Geometry: final body of the model. Coordinates: model frame, mm. Coordinates: 2 decimals unless noted, no trailing zeros. Write each loop counter-clockwise with the first axis right and the second up, starting at its lowest first coordinate (ties: lowest second). Pieces come first, ordered by that corner, then holes.
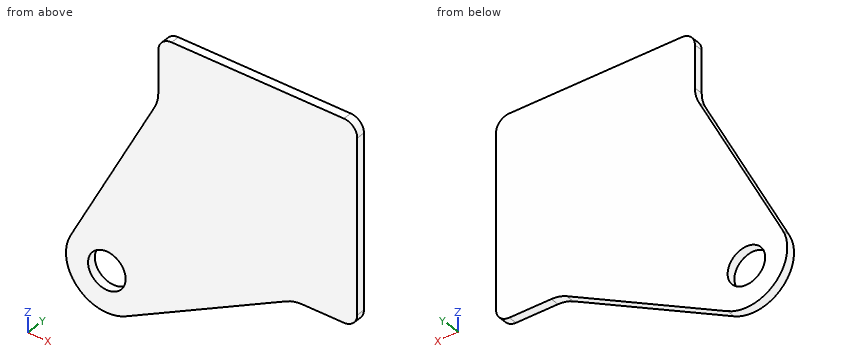
Autodesk Inventor part; units mm, degrees
ref_plane "YZ Plane" through (0, 0, 0) normal (1, 0, 0) x (0, 1, 0)
ref_plane "XZ Plane" through (0, 0, 0) normal (0, 1, 0) x (-1, 0, 0)
ref_plane "XY Plane" through (0, 0, 0) normal (0, 0, 1) x (1, 0, 0)
sketch "Sketch1" plane through (0, 0, 0) normal (0, 1, 0) x (-1, 0, 0)
  line L0 (40, 40) -> (-40, 40) construction
  line L1 (-40, 40) -> (-40, -40) construction
  line L2 (-40, -40) -> (40, -40) construction
  line L3 (40, -40) -> (40, 40) construction
  line L4 (-40, 40) -> (40, -40) construction
  line L5 (0, 40) -> (0, -40) construction
  line L6 (-45, -45) -> (-45, 0)
  line L7 (-20, -45) -> (-45, -45)
  arc A0 (59.7253, -84.6853) -> (84.6853, -59.7253) centre (68.2843, -68.2843) ccw
  circle A1 centre (68.2843, -68.2843) radius 8.5
  line L8 (59.7253, -84.6853) -> (-13.0603, -46.7019)
  arc A2 (-13.0603, -46.7019) -> (-20, -45) centre (-20, -60) ccw
  arc A3 (84.6853, -59.7253) -> (59.7253, -84.6853) centre (68.2843, -68.2843) ccw construction
  line L9 (84.6853, -59.7253) -> (46.7019, 13.0603)
  line L10 (-45, 0) -> (-45, 45)
  line L11 (-45, 45) -> (45, 45)
  line L12 (45, 45) -> (45, 20)
  arc A4 (45, 20) -> (46.7019, 13.0603) centre (60, 20) ccw
  line L13 (40, 0) -> (45, 0) construction
  line L14 (0, 40) -> (0, 45) construction
  line L15 (-40, 0) -> (-45, 0) construction
  point P0 (0, 0)
  point P1 (0, 0)
  point P2 (0, 0)
  dimension "d2" = 80
  dimension "d3" = 80
  dimension "d29" = 5
  dimension "d30" = 17
  dimension "d31" = 10
  dimension "d32" = 40
  dimension "d34" = 5
  dimension "d35" = 15
  dimension "d36" = 25
extrude "Plate1" add sketch "Sketch1" along normal blind 4
fillet "Corner Round3" radius 6 3 edges at (-45, 2, 45) (45, 2, 45) (45, 2, -45)
equation "\"d34\" = d29"
equation "\"d6\" = Thickness"
properties part number "MSC 901 BASE PLATE" material "Stainless Steel"
Item 1: Section B-B, the plane x = -66. Output: boundary loops of the cut face in (y, z), plus the area to 3 significant figures.
Derived:
outline: (0, -86.64) - (4, -86.64) - (4, -76.47) - (0, -76.47) - close; (0, -60.1) - (4, -60.1) - (4, -23.92) - (0, -23.92) - close
area: 185 mm2
Item 2: Section D-D, the plane z = 26. Output: boundary loops of the cut face in (x, y).
Derived:
outline: (-45, 0) - (45, 0) - (45, 4) - (-45, 4) - close
Item 3: Material intervals for probe 1 along X at (y, z) = (3.5, -67.5); probe 2 along Z at (x, y) = (26, 0.55); probe 3 along X at (y, z) = (1.4, -62), sorted ascending.
Derived:
probe 1: x = -86.77 to -76.75, -59.82 to -26.79
probe 2: z = -45 to 45
probe 3: x = -85.68 to -74.01, -62.56 to -16.25
Item 4: Section C-C, the plane y = 2.4. Output: boundary loops of the cut face in (x, z), plus the area to 3 significant figures.
Derived:
outline: (-84.69, -59.73) arc R18.5 ccw to (-59.73, -84.69) - (13.06, -46.7) arc R15 cw to (20, -45) - (39, -45) arc R6 ccw to (45, -39) - (45, 39) arc R6 ccw to (39, 45) - (-39, 45) arc R6 ccw to (-45, 39) - (-45, 20) arc R15 cw to (-46.7, 13.06) - close; hole circle Ø17 at (-68.28, -68.28)
area: 11,300 mm2
Item 5: Section A-A, the plane z = -73.5. Output: boundary loops of the cut face in (x, y), plus the area to 3 significant figures.
Derived:
outline: (-86.03, 0) - (-75, 0) - (-75, 4) - (-86.03, 4) - close; (-61.57, 0) - (-38.29, 0) - (-38.29, 4) - (-61.57, 4) - close
area: 137 mm2
Item 6: Pin query (flat end, axial travel): pin 1 (2 mm diameter, centred on y = 1.5, z = 30, fed in from -X). Return the tip coordinate at first contact, or that it passes through.
Derived:
pin 1: stops at x = -45
